Source: CAD feature listing. Evaluate the final solid. Frame: model axes, mm. Face numbers are marked on the shaded views. Give positions to 0.01 mm unless a question says otherwise; leave off trailing zeros. Loops run counter-clockwise (first coordinate to the right, second up) from the corner with the lowest first, then second, coordinate; pieces in that order, holes last.
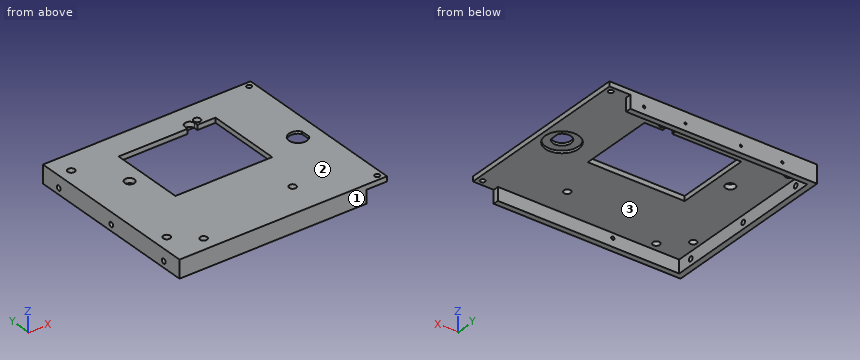
from build123d import *

# Parameters (mm, degrees)
COPYSKETCH010_W   = 150
COPYSKETCH010_H   = 130
COPYSKETCH010_R   = 2.5
COPYSKETCH010_R_2 = 3.5
COPYSKETCH010_R_3 = 1.75
PAD_DEPTH         = 3.5
PAD001_DEPTH      = 13
SKETCH001_R       = 1.75
POCKET_DEPTH      = 5
SKETCH002_R       = 1.15
POCKET001_DEPTH   = 2.5
SKETCH003_R       = 0.875
SKETCH003_R_2     = 0.75
POCKET002_DEPTH   = 2.5
SKETCH004_R       = 12
POCKET003_DEPTH   = 1.75


with BuildPart() as part:
    # CopySketch010 → Pad (new body)
    with BuildSketch(Plane(origin=(0, 0, 0), x_dir=(-1, 0, 0), z_dir=(0, 0, -1))):
        with Locations((-75, 0)):
            Rectangle(COPYSKETCH010_W, COPYSKETCH010_H)
        with Locations((-100, 50)):
            Circle(COPYSKETCH010_R, mode=Mode.SUBTRACT)
        with Locations((-100, -41)):
            Circle(COPYSKETCH010_R, mode=Mode.SUBTRACT)
        with Locations((-9, -41)):
            Circle(COPYSKETCH010_R, mode=Mode.SUBTRACT)
        with Locations((-9, 50)):
            Circle(COPYSKETCH010_R, mode=Mode.SUBTRACT)
        with Locations((-28.79, 20.377)):
            Circle(COPYSKETCH010_R_2, mode=Mode.SUBTRACT)
        with Locations((-146, 61)):
            Circle(COPYSKETCH010_R_3, mode=Mode.SUBTRACT)
        with Locations((-146, -61)):
            Circle(COPYSKETCH010_R_3, mode=Mode.SUBTRACT)
        with Locations((-25, -55)):
            Circle(COPYSKETCH010_R, mode=Mode.SUBTRACT)
        with BuildLine():
            Line((-40, -8.35), (-110, -8.35))
            Line((-110, -8.35), (-110, 45.65))
            Line((-110, 45.65), (-96.908, 45.65))
            Line((-96.908, 48.264), (-96.908, 45.65))
            ThreePointArc((-89.908002, 48.26), (-93.406, 51.763999), (-96.908, 48.264))
            Line((-89.908002, 48.26), (-89.908002, 45.65))
            Line((-89.908002, 45.65), (-40, 45.65))
            Line((-40, 45.65), (-40, -8.35))
        make_face(mode=Mode.SUBTRACT)
        with BuildLine():
            ThreePointArc((-140.5, -3.464102), (-128.5, 0), (-140.5, 3.464102))
            Line((-140.5, -3.464102), (-140.5, 3.464102))
        make_face(mode=Mode.SUBTRACT)
    extrude(amount=PAD_DEPTH)

    # Sketch (on Face23 of Pad) → Pad001 (join)
    with BuildSketch(Plane.XY):
        Polygon((135, 65), (135, 61), (4, 61), (4, -61), (135, -61), (135, -65), (0, -65), (0, 65), align=None)
    extrude(amount=-PAD001_DEPTH)

    # Sketch001 → Pocket (cut)
    with BuildSketch(Plane.YZ):
        with Locations((0, -8.5)):
            Circle(SKETCH001_R)
        with Locations((50, -8.5)):
            Circle(SKETCH001_R)
        with Locations((-50, -8.5)):
            Circle(SKETCH001_R)
    extrude(amount=POCKET_DEPTH, mode=Mode.SUBTRACT)

    # Sketch002 → Pocket001 (cut, symmetric)
    with BuildSketch(Plane.XZ.offset(60)):
        with Locations((52, -7)):
            Circle(SKETCH002_R)
    extrude(amount=POCKET001_DEPTH, both=True, mode=Mode.SUBTRACT)

    # Sketch003 → Pocket002 (cut, symmetric)
    with BuildSketch(Plane.XZ.offset(-65)):
        with Locations((25, -8)):
            Circle(SKETCH003_R)
        with Locations((125, -8)):
            Circle(SKETCH003_R)
        with Locations((95, -8)):
            Circle(SKETCH003_R_2)
        with Locations((55, -8)):
            Circle(SKETCH003_R_2)
    extrude(amount=POCKET002_DEPTH, both=True, mode=Mode.SUBTRACT)

    # Sketch004 → Pocket003 (cut)
    with BuildSketch(Plane.XY.offset(-3.5)):
        with Locations((135, 0)):
            Circle(SKETCH004_R)
    extrude(amount=POCKET003_DEPTH, mode=Mode.SUBTRACT)


solid = part.part
1) Ray query, probe 1 along Y at (x, z) = (1.6, -8.5); probe 2 along Y at (x, z) = (9, -1.9); probe 3 along X at (y, z) = (0, -0.35). Return the intervals inside material, ascending.
Checks:
probe 1: y = -65 to -51.75, -48.25 to -1.75, 1.75 to 48.25, 51.75 to 65
probe 2: y = -65 to -43.5, -38.5 to 47.5, 52.5 to 65
probe 3: x = 0 to 40, 110 to 128.5, 140.5 to 150
2) Contact query for flat-ended pins moving along their axis: P1, Ø4.5, axis at y = 63, z = -10, coming from the +X side; P2, Ø2, axis at x = 40.5, y = -2.5, coming from the -Z side; P3, Ø4.5, axis at x = 100, y = -41, coming from the -Z side; P4, Ø1.2, axis at x = 55, z = -8, coming from the +Y side. Output: stop coordinate, or through.
Checks:
P1: stops at x = 135
P2: stops at z = -3.5
P3: passes through
P4: stops at y = 62.5
3) Pull-direction query (Y, two-part tool) for the marked faces 1, 2 and 3; classes: released by +Y, released by -Y, zero draft, split by the parting line, or undercut.
Checks:
face 1: released by -Y
face 2: zero draft
face 3: undercut
4) Cut plane B-B (x = 38). Return loops of the section in (y, z), and give its area (3 significant figures).
Checks:
outline: (-65, -13) - (-61, -13) - (-61, -3.5) - (61, -3.5) - (61, -13) - (65, -13) - (65, 0) - (-65, 0) - close
area: 531 mm2
5) Cut plane A-A (y = -55). Return loops of the section in (x, z), and give its area (4 significant figures).
Checks:
outline: (0, -13) - (4, -13) - (4, -3.5) - (22.5, -3.5) - (22.5, 0) - (0, 0) - close; (27.5, -3.5) - (150, -3.5) - (150, 0) - (27.5, 0) - close
area: 545.5 mm2
6) Cut plane D-D (x = 131). Return loops of the section in (y, z).
Checks:
outline: (-65, -13) - (-61, -13) - (-61, -3.5) - (-11.31, -3.5) - (-11.31, -1.75) - (-5.12, -1.75) - (-5.12, 0) - (-65, 0) - close; (5.12, -1.75) - (11.31, -1.75) - (11.31, -3.5) - (61, -3.5) - (61, -13) - (65, -13) - (65, 0) - (5.12, 0) - close
7) Cut plane C-C (y = -36). Return loops of the section in (x, z), and give its area (3 significant figures).
Checks:
outline: (0, -13) - (4, -13) - (4, -3.5) - (150, -3.5) - (150, 0) - (0, 0) - close
area: 563 mm2
